Geometry check sheet. Reference: the model listing, model coordinates, mm. Coordinates: 2 decimals unless noted, no trailing zeros. Write each loop counter-clockwise with the first axis right and the second up, starting at its lowest first coordinate (ties: lowest second). Pieces come first, ordered by that corner, then holes. Notation, with made-up numbers: M 83.5,63.5 L 136.5,63.5 A17 cw 136.5,87.5 Z; hole C -7.75,-13 d10. An arc over 180 degrees is marked long. Answer as a JSON object with one key per item and string values. Group by question number.
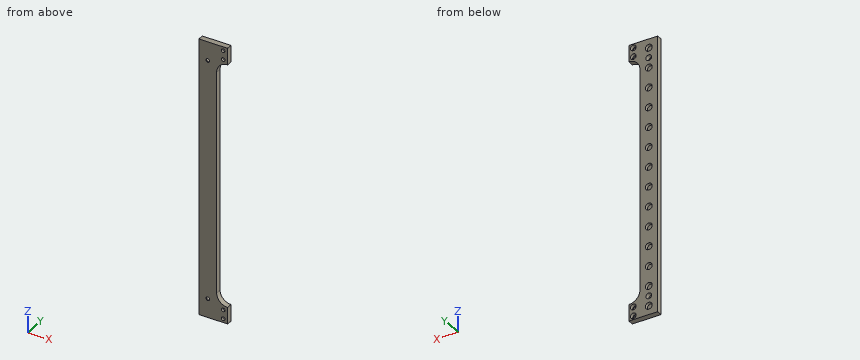
```python
from build123d import *

# Parameters (mm, degrees)
SKETCH1_W           = 16
SKETCH1_H           = 250
BOSS_EXTRUDE1_DEPTH = 5
SKETCH2_R           = 3.1
CUT_EXTRUDE1_DEPTH  = 2.8
SKETCH4_W           = 10
SKETCH4_H           = 15
BOSS_EXTRUDE2_DEPTH = 5
CUT_EXTRUDE2_REACH  = 253.398
SKETCH5_R           = 1.65
SKETCH6_R           = 2.6
CUT_EXTRUDE3_DEPTH  = 3
FILLET1_R           = 10
SKETCH8_R           = 2.6
CUT_EXTRUDE4_DEPTH  = 4


with BuildPart() as part:
    # Sketch1 → Boss-Extrude1 (new body)
    with BuildSketch(Plane(origin=(0, 0, 0), x_dir=(1, 0, 0), z_dir=(0, 1, 0))):
        with Locations((8, 125)):
            Rectangle(SKETCH1_W, SKETCH1_H)
    extrude(amount=BOSS_EXTRUDE1_DEPTH)

    # Sketch2 → Cut-Extrude1 (cut)
    with BuildSketch(Plane(origin=(0, 5, 0), x_dir=(1, 0, 0), z_dir=(0, 1, 0))):
        with Locations(Location((8, 242, 0), (0, 0, 270))):
            Circle(SKETCH2_R)
        with Locations(Location((8, 224, 0), (0, 0, 270))):
            Circle(SKETCH2_R)
        with Locations(Location((8, 206, 0), (0, 0, 270))):
            Circle(SKETCH2_R)
        with Locations(Location((8, 188, 0), (0, 0, 270))):
            Circle(SKETCH2_R)
        with Locations(Location((8, 170, 0), (0, 0, 270))):
            Circle(SKETCH2_R)
        with Locations(Location((8, 152, 0), (0, 0, 270))):
            Circle(SKETCH2_R)
        with Locations(Location((8, 134, 0), (0, 0, 270))):
            Circle(SKETCH2_R)
        with Locations(Location((8, 116, 0), (0, 0, 270))):
            Circle(SKETCH2_R)
        with Locations(Location((8, 98, 0), (0, 0, 270))):
            Circle(SKETCH2_R)
        with Locations(Location((8, 80, 0), (0, 0, 270))):
            Circle(SKETCH2_R)
        with Locations(Location((8, 62, 0), (0, 0, 270))):
            Circle(SKETCH2_R)
        with Locations(Location((8, 44, 0), (0, 0, 270))):
            Circle(SKETCH2_R)
        with Locations(Location((8, 26, 0), (0, 0, 270))):
            Circle(SKETCH2_R)
        with Locations(Location((8, 8, 0), (0, 0, 270))):
            Circle(SKETCH2_R)
    extrude(amount=-CUT_EXTRUDE1_DEPTH, mode=Mode.SUBTRACT)

    # Sketch4 → Boss-Extrude2 (add)
    with BuildSketch(Plane(origin=(0, 5, 0), x_dir=(1, 0, 0), z_dir=(0, 1, 0))):
        with Locations((21, 7.5)):
            Rectangle(SKETCH4_W, SKETCH4_H)
        with Locations((21, 242.5)):
            Rectangle(SKETCH4_W, SKETCH4_H)
    extrude(amount=-BOSS_EXTRUDE2_DEPTH)

    # Sketch5 → Cut-Extrude2 (cut, up to next)
    with BuildSketch(Plane.XZ, mode=Mode.PRIVATE) as cut_extrude2_sk1:
        with Locations(Location((22, -3.5, 0), (0, 0, 270))):
            Circle(SKETCH5_R)
    cut_extrude2_tool1 = extrude(cut_extrude2_sk1.sketch, amount=-CUT_EXTRUDE2_REACH, mode=Mode.PRIVATE) & part.part
    # Sketch5 → Cut-Extrude2 (cut, up to next)
    with BuildSketch(Plane.XZ, mode=Mode.PRIVATE) as cut_extrude2_sk2:
        with Locations(Location((22, -11.5, 0), (0, 0, 270))):
            Circle(SKETCH5_R)
    cut_extrude2_tool2 = extrude(cut_extrude2_sk2.sketch, amount=-CUT_EXTRUDE2_REACH, mode=Mode.PRIVATE) & part.part
    # Sketch5 → Cut-Extrude2 (cut, up to next)
    with BuildSketch(Plane.XZ, mode=Mode.PRIVATE) as cut_extrude2_sk3:
        with Locations(Location((22, -238.5, 0), (0, 0, 270))):
            Circle(SKETCH5_R)
    cut_extrude2_tool3 = extrude(cut_extrude2_sk3.sketch, amount=-CUT_EXTRUDE2_REACH, mode=Mode.PRIVATE) & part.part
    # Sketch5 → Cut-Extrude2 (cut, up to next)
    with BuildSketch(Plane.XZ, mode=Mode.PRIVATE) as cut_extrude2_sk4:
        with Locations(Location((22, -246.5, 0), (0, 0, 270))):
            Circle(SKETCH5_R)
    cut_extrude2_tool4 = extrude(cut_extrude2_sk4.sketch, amount=-CUT_EXTRUDE2_REACH, mode=Mode.PRIVATE) & part.part
    # Sketch5 → Cut-Extrude2 (cut, up to next)
    with BuildSketch(Plane.XZ, mode=Mode.PRIVATE) as cut_extrude2_sk5:
        with Locations(Location((8, -17, 0), (0, 0, 270))):
            Circle(SKETCH5_R)
    cut_extrude2_tool5 = extrude(cut_extrude2_sk5.sketch, amount=-CUT_EXTRUDE2_REACH, mode=Mode.PRIVATE) & part.part
    # Sketch5 → Cut-Extrude2 (cut, up to next)
    with BuildSketch(Plane.XZ, mode=Mode.PRIVATE) as cut_extrude2_sk6:
        with Locations(Location((8, -233, 0), (0, 0, 270))):
            Circle(SKETCH5_R)
    cut_extrude2_tool6 = extrude(cut_extrude2_sk6.sketch, amount=-CUT_EXTRUDE2_REACH, mode=Mode.PRIVATE) & part.part
    add(cut_extrude2_tool1.solids().sort_by_distance((22, 0, -3.5))[0], mode=Mode.SUBTRACT)
    add(cut_extrude2_tool2.solids().sort_by_distance((22, 0, -11.5))[0], mode=Mode.SUBTRACT)
    add(cut_extrude2_tool3.solids().sort_by_distance((22, 0, -238.5))[0], mode=Mode.SUBTRACT)
    add(cut_extrude2_tool4.solids().sort_by_distance((22, 0, -246.5))[0], mode=Mode.SUBTRACT)
    add(cut_extrude2_tool5.solids().sort_by_distance((8, 0, -17))[0], mode=Mode.SUBTRACT)
    add(cut_extrude2_tool6.solids().sort_by_distance((8, 0, -233))[0], mode=Mode.SUBTRACT)

    # Sketch6 → Cut-Extrude3 (cut)
    with BuildSketch(Plane(origin=(0, 5, 0), x_dir=(1, 0, 0), z_dir=(0, 1, 0))):
        with Locations(Location((22, 246.5, 0), (0, 0, 270))):
            Circle(SKETCH6_R)
        with Locations(Location((22, 238.5, 0), (0, 0, 270))):
            Circle(SKETCH6_R)
        with Locations(Location((22, 11.5, 0), (0, 0, 270))):
            Circle(SKETCH6_R)
        with Locations(Location((22, 3.5, 0), (0, 0, 270))):
            Circle(SKETCH6_R)
        with Locations(Location((8, 233, 0), (0, 0, 270))):
            Circle(SKETCH6_R)
        with Locations(Location((8, 17, 0), (0, 0, 270))):
            Circle(SKETCH6_R)
    extrude(amount=-CUT_EXTRUDE3_DEPTH, mode=Mode.SUBTRACT)

    # Fillet1
    fillet1_edges = [part.edges().sort_by_distance(p)[0] for p in [
        (16, 2.5, -235),
        (16, 2.5, -15),
    ]]
    fillet(fillet1_edges, radius=FILLET1_R - 0.0001)  # a hair under: the kernel refuses the full size

    # Sketch8 → Cut-Extrude4 (cut)
    with BuildSketch(Plane(origin=(0, 5, 0), x_dir=(1, 0, 0), z_dir=(0, 1, 0))):
        with Locations(Location((8, 233, 0), (0, 0, 270))):
            Circle(SKETCH8_R)
        with Locations(Location((8, 17, 0), (0, 0, 270))):
            Circle(SKETCH8_R)
    extrude(amount=-CUT_EXTRUDE4_DEPTH, mode=Mode.SUBTRACT)


solid = part.part
```
1) Section check A-A (y = 3.1). State how many separate pieces and enclosed holes the cut face has, then the cut area to 3 significant figures.
2) Section check C-C (z = -163). Record the cut outline in (x, y).
3) Material ranges on probe 1 along Z at (x, y) = (6, 2.05); probe 2 along X at (y, z) = (4.05, -62); probe 3 along Z at (x, y) = (9, 1.2), recorded low to high. Write a range as [from, to].
4) Go/stop test with flat-tipped pins: pin 1 Ø2 at (x, z) = (22, -3.5) entering from +Y; pin 2 Ø5.5 at (x, z) = (8, -8) entering from +Y. Record where each tip stops, or that it passes through.
5) Section check B-B (z = -206). Record the cut outline in (x, y), then the cut area to 3 significant figures.
Entries:
{
 "1": {"separate pieces": "1", "enclosed holes": "20", "area": "3,790 mm^2"},
 "2": {"outline": "M 0,0 L 16,0 L 16,5 L 0,5 Z"},
 "3": {"probe 1": "[-250, -234.66], [-231.34, -18.66], [-15.34, 0]", "probe 2": "[0, 4.9], [11.1, 16]", "probe 3": "[-250, -235.4], [-230.6, -19.4], [-14.6, 0]"},
 "4": {"pin 1": "through", "pin 2": "y = 2.2"},
 "5": {"outline": "M 0,0 L 16,0 L 16,5 L 11.1,5 L 11.1,2.2 L 4.9,2.2 L 4.9,5 L 0,5 Z", "area": "62.6 mm^2"}
}
